Read the model definition and answer for the solid it produces. Units are mm, in the model's axes. A direction names the side the tool comes from. Give positions to 0.01 mm unless a question says otherwise; leave off trailing zeros. Order: outer loops, then holes, each group sorted by start corner. A loop starts at its lowest first (then second) coordinate and runs counter-clockwise, first axis right, second up.
```python
from build123d import *

# Parameters (mm, degrees)
SKETCH1_W           = 500
SKETCH1_H           = 500
BOSS_EXTRUDE1_DEPTH = 20
SKETCH1_3_W         = 20
SKETCH1_3_H         = 40
SKETCH1_3_W_2       = 40
SKETCH1_3_H_2       = 20
BOSS_EXTRUDE2_DEPTH = 40
SKETCH5_R           = 10
CUT_EXTRUDE1_DEPTH  = 526.071423713
SKETCH6_R           = 10
CUT_EXTRUDE2_DEPTH  = 526.071423713


with BuildPart() as part:
    # Sketch1 → Boss-Extrude1 (new body)
    with BuildSketch(Plane(origin=(0, 0, 0), x_dir=(1, 0, 0), z_dir=(0, 1, 0))):
        Rectangle(SKETCH1_W, SKETCH1_H)
    extrude(amount=-BOSS_EXTRUDE1_DEPTH)

    # Sketch1<3> → Boss-Extrude2 (add)
    with BuildSketch(Plane(origin=(0, 0, 0), x_dir=(1, 0, 0), z_dir=(0, 1, 0))):
        with Locations((-200, -50)):
            Rectangle(SKETCH1_3_W, SKETCH1_3_H)
        with Locations((-50, 200)):
            Rectangle(SKETCH1_3_W_2, SKETCH1_3_H_2)
        with Locations((200, 50)):
            Rectangle(SKETCH1_3_W, SKETCH1_3_H)
        with Locations((50, -200)):
            Rectangle(SKETCH1_3_W_2, SKETCH1_3_H_2)
    extrude(amount=BOSS_EXTRUDE2_DEPTH)

    # Sketch5 → Cut-Extrude1 (cut, through all)
    with BuildSketch(Plane(origin=(0, 0, -210), x_dir=(-1, 0, 0), z_dir=(0, 0, -1))):
        with Locations((50, 20)):
            Circle(SKETCH5_R)
    extrude(amount=-CUT_EXTRUDE1_DEPTH, mode=Mode.SUBTRACT)

    # Sketch6 → Cut-Extrude2 (cut, through all)
    with BuildSketch(Plane(origin=(210, 0, 0), x_dir=(0, 0, -1), z_dir=(1, 0, 0))):
        with Locations((50, 20)):
            Circle(SKETCH6_R)
    extrude(amount=-CUT_EXTRUDE2_DEPTH, mode=Mode.SUBTRACT)

    # Sketch7 → Revolve1 (revolve)
    with BuildSketch(Plane(origin=(0, 0, 0), x_dir=(0, 0, -1), z_dir=(1, 0, 0))):
        Polygon((0, 0), (0, 140), (10, 130), (10, 0), align=None)
    revolve(axis=Axis((0, 0, 0), (0, 1, 0)))


solid = part.part
```
1) Consider L1, parallel to Y at x = 201, z = -50; L2, parallel to Y at x = -21.5, z = -208.5; L3, parallel to Z at x = -42.5, y = 29.5. Determine where each line is inside the solid, lowest interval first.
Final values:
L1: y = -20 to 10, 30 to 40
L2: y = -20 to 0
L3: z = -210 to -190
2) The part is cut by section A-A on y = 20. Determine the outline of the cut face in (x, z), and give its area (3 significant figures).
Final values:
outline: (-210, 30) - (-190, 30) - (-190, 70) - (-210, 70) - close; (-70, -210) - (-60, -210) - (-60, -190) - (-70, -190) - close; (-40, -210) - (-30, -210) - (-30, -190) - (-40, -190) - close; circle Ø20 at (0, 0); (30, 190) - (70, 190) - (70, 210) - (30, 210) - close; (190, -70) - (210, -70) - (210, -60) - (190, -60) - close; (190, -40) - (210, -40) - (210, -30) - (190, -30) - close
area: 2,710 mm2
3) The part is cut by section B-B on z = -50. Determine the outline of the cut face in (x, y).
Final values:
outline: (-250, -20) - (250, -20) - (250, 0) - (210, 0) - (210, 10) - (190, 10) - (190, 0) - (-250, 0) - close; (190, 30) - (210, 30) - (210, 40) - (190, 40) - close
4) A tool of negligible diameter and unlimited length cuts with its end or side. For faces 1 (the face through (50, 20, 210)), 2 (the face through (30, 20, 200)), 3 (the face through (50, 20, 190)), 4 (the face through (-190, 20, 50)), from which of +Z, -Z, +X, -X, +Y, -Y can it reach the whole face along a straight path? Write none if from no direction.
Final values:
face 1: +Z, +X, -X, +Y
face 2: +Z, -Z, -X, +Y
face 3: -Z, +X, -X, +Y
face 4: +Z, -Z, +X, +Y
5) The part is cut by section C-C on y = 120.5. Determine the outline of the cut face in (x, z).
Final values:
outline: circle Ø20 at (0, 0)
6) Given pin 1 (1 mm diameter, centred on x = 1, y = 36.5, fed in from -Z); pin 2 (2 mm diameter, centred on x = -199, y = 13.5, fed in from -Z); pin 3 (6 mm diameter, centred on y = 18.5, z = -199, fed in from -X), each flat-ended and moving along its own axis, determine where each tip first touches the part or whether it passes through.
Final values:
pin 1: stops at z = -9.99
pin 2: stops at z = 30
pin 3: stops at x = -70
7) The part is cut by section D-D on x = -16. Determine the outline of the cut face in (y, z).
Final values:
outline: (-20, -250) - (0, -250) - (0, 250) - (-20, 250) - close
